Can you work these out from the model? Positions are in its coordinate system, mm. Face numbers are marked on the shaded views. A direction names the side the tool comes from. Round coordinates to 2 decimals unless told otherwise and drop trailing zeros. Write each loop counter-clockwise with the first axis right and the second up, starting at its lowest first coordinate (ties: lowest second). Pieces come first, ordered by that corner, then holes. Notation, with made-up numbers: (4.25, 34) -> (17.25, 34) arc R8 cw to (17.25, 47) -> close; hole circle Ø10 at (86, -14). An arc over 180 degrees is marked (long way). Use CSV: the item, a comma, the result in double quotes.
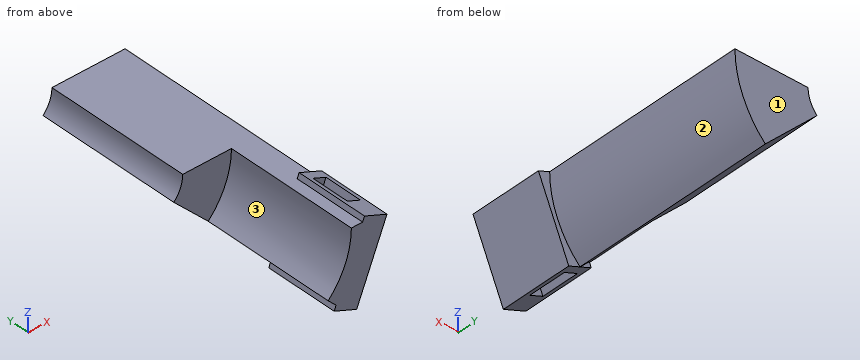
```python
from build123d import *

# Parameters (mm, degrees)
REVOLVE1_ANGLE      = 45
SKETCH2_W           = 32.528091751
SKETCH2_H           = 30
BOSS_EXTRUDE1_DEPTH = 5
SKETCH3_W           = 5.8
SKETCH3_H           = 15.8
CUT_EXTRUDE1_DEPTH  = 43.413800206


with BuildPart() as part:
    # Sketch1 → Revolve1 (revolve)
    with BuildSketch(Plane.XY):
        Polygon((0, 0), (0, 60), (30, 60), (30, -55), (20, -55), (20, 0), align=None)
    revolve(axis=Axis((-12.5, 0, 0), (0, 1, 0)), revolution_arc=REVOLVE1_ANGLE)

    # Sketch2 → Boss-Extrude1 (add, symmetric)
    with BuildSketch(Plane(origin=(25.606601718, 0, -10.606601718), x_dir=(0.382683432, 0, 0.923879533), z_dir=(-0.923879533, 0, 0.382683432))):
        with Locations((-4.783542905, -40)):
            Rectangle(SKETCH2_W, SKETCH2_H)
    extrude(amount=BOSS_EXTRUDE1_DEPTH, both=True)

    # Sketch3 → Cut-Extrude1 (cut, through all)
    with BuildSketch(Plane(origin=(4.393398282, 0, 10.606601718), x_dir=(0.923879533, 0, -0.382683432), z_dir=(0.382683432, 0, 0.923879533))):
        with Locations((27.716385975, -37.1)):
            Rectangle(SKETCH3_W, SKETCH3_H)
    extrude(amount=-CUT_EXTRUDE1_DEPTH, mode=Mode.SUBTRACT)


solid = part.part
```
Q1. Please list where these lines run through material, in increasing order: probe 1 along Y at (x, z) = (18.5, -29); probe 2 along Y at (x, z) = (14.5, -13); probe 3 along X at (y, z) = (36, -0.5).
Resolved:
probe 1,"y = -55 to -45, -29.2 to 60"
probe 2,"y = 0 to 60"
probe 3,"x = -0.01 to 30"
Q2. Suppose I cut it at D-D (x = 23.5). Write out the boundary of the cut face in (y, z), and give its area (3 significant figures).
Resolved:
outline,"(-55, -28.76) -> (-25, -28.76) -> (-25, -22.59) -> (60, -22.59) -> (60, 0) -> (-55, 0) -> close; hole (-45, -23.27) -> (-29.2, -23.27) -> (-29.2, -8.11) -> (-45, -8.11) -> close"
area,"2,540 mm^2"
Q3. Suppose I cut it at A-A (y = -32.5). Write out the boundary of the cut face in (x, z).
Resolved:
outline,"(10.48, -22.98) -> (13.73, -26.23) -> (12.93, -28.14) -> (14.87, -28.94) -> (27.32, 1.11) -> (25.38, 1.91) -> (24.59, 0) -> (20, 0) arc R32.5 cw to start; (20.23, -31.16) -> (22.17, -31.97) -> (34.62, -1.91) -> (32.68, -1.11) -> close"
Q4. Suppose I cut it at B-B (z = -21.5). Write out the boundary of the cut face in (x, y), and give its area (3 significant figures).
Resolved:
outline,"(9, 0) -> (11.87, 0) -> (11.87, -55) -> (26.51, -55) -> (26.51, -25) -> (24.16, -25) -> (24.16, 60) -> (9, 60) -> close; hole (17.96, -45) -> (24.23, -45) -> (24.23, -29.2) -> (17.96, -29.2) -> close"
area,"1,560 mm^2"
Q5. On a 3-axis mill with a long thin cutter (end or side, diameter ignored), from which of +Z, -Z, +X, -X, +Y, -Y can I reach the whole of each face in a straight line? I mean the marked faces 1, 2 and 3. Say none if no direction works.
Resolved:
face 1,"+Z, -Z, +X, -X, +Y"
face 2,"-Z, +X, +Y"
face 3,"+Z, -X, -Y"
Q6. Will these pins go through, and if not, where does the flat tip stop? P1, Ø5, axis at x = 29, z = -19.5, coming from the +Y side; P2, Ø8, axis at y = 42.5, z = -4.5, coming from the -X side; P3, Ø2, axis at y = 45.5, z = -21.5, coming from the +X side.
Resolved:
P1,"stops at y = -25"
P2,"stops at x = -3.33"
P3,"stops at x = 24.73"
Q7. Suppose I cut it at C-C (y = -47). Write out the boundary of the cut face in (x, z), and give its area (3 significant figures).
Resolved:
outline,"(10.48, -22.98) -> (13.73, -26.23) -> (12.93, -28.14) -> (22.17, -31.97) -> (34.62, -1.91) -> (25.38, 1.91) -> (24.59, 0) -> (20, 0) arc R32.5 cw to start"
area,"397 mm^2"
